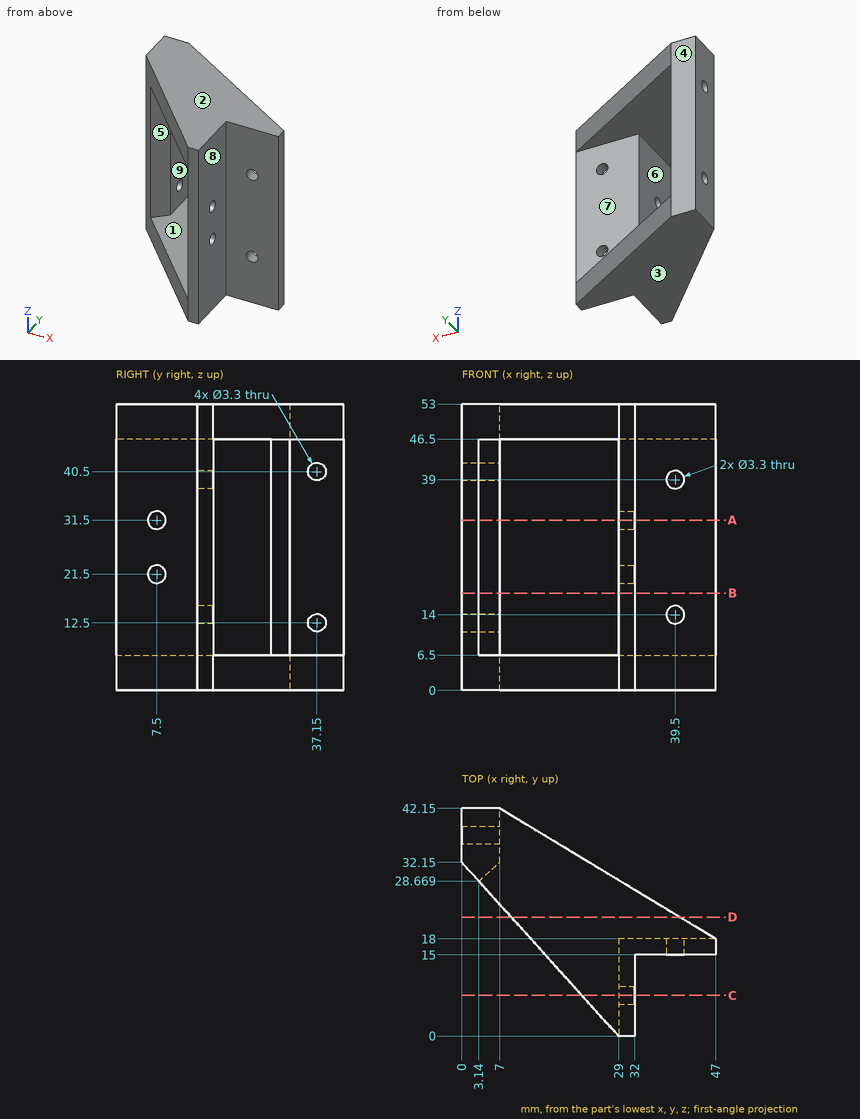
Study the drawing (mm; zero at the part's minimum x, y, z) and answer. A direction names the side the tool comes from. Give positions to 0.01 mm unless a question says otherwise; leave off trailing zeros. Loops run counter-clockwise (first coordinate to the right, second up) from the corner with the lowest first, then second, coordinate; pieces in that order, holes last. Notation, with made-up numbers: (83, 67) - (93, 67) arc R16 ccw to (93, 90) - close; hole circle Ø7 at (12, -40). An arc over 180 degrees is marked (long way). One line per question, with ' | ' between items.
(1) A tool of negligible diameter and unlimited length cuts with its end or side. For the marked faces 5, 6, 7, 8 and 9, from which of +Z, -Z, +X, -X, +Y, -Y can it reach the whole face along a straight path? Write none if from no direction.
Recorded:
face 5: +X, -Y | face 6: -X, +Y, -Y | face 7: +X, -X, +Y | face 8: +Z, -Z, +X, -Y | face 9: +X, +Y, -Y
(2) Each of these flat-tipped pins is pushed along its axis until it touches: pin 1 Ø2 at (y, z) = (37.15, 12.5) entering from -X; pin 2 Ø14.5 at (y, z) = (7, 24) entering from -X; pin 3 Ø20 at (x, z) = (42, 30.5) entering from +Y; pin 4 Ø5.5 at (x, z) = (39.5, 39) entering from -Y. Where does it stop, or does it pass through?
Recorded:
pin 1: passes through | pin 2: stops at x = 29 | pin 3: stops at y = 18 | pin 4: stops at y = 15
(3) The part is cut by section B-B (z = 18). Write down the section's boundary in (x, y).
Recorded:
outline: (0, 32.15) - (3.14, 28.67) - (7, 32.15) - (7, 42.15) - (0, 42.15) - close; (29, 0) - (32, 0) - (32, 15) - (47, 15) - (47, 18) - (29, 18) - close
(4) Straight lines are drawn through the part: probe 1 along Z at (x, y) = (25, 15); probe 2 along Z at (x, y) = (39.5, 15.6); probe 3 along Z at (x, y) = (29.75, 7.5). For each, find the intervals that lie inside material, in ascending order.
Recorded:
probe 1: z = 0 to 6.5, 46.5 to 53 | probe 2: z = 0 to 12.35, 15.65 to 37.35, 40.65 to 53 | probe 3: z = 0 to 19.85, 23.15 to 29.85, 33.15 to 53
(5) The mould has two halves that part along Z. Classify the marked faces 1, 2, 3 and 4: +Z half, -Z half, draft (parallel to the pull), parting line (faces both ways), or undercut.
Recorded:
face 1: undercut | face 2: +Z half | face 3: -Z half | face 4: draft
(6) The part is cut by section C-C (y = 7.5). Count the separate pieces of the cut face and the enclosed holes in it, then the cut area to 3 significant figures.
Recorded:
separate pieces: 3 | enclosed holes: 0 | area: 227 mm²
(7) The part is cut by section A-A (z = 31.5). Write down the section's boundary in (x, y).
Recorded:
outline: (0, 32.15) - (3.14, 28.67) - (7, 32.15) - (7, 42.15) - (0, 42.15) - close; (29, 0) - (32, 0) - (32, 5.85) - (29, 5.85) - close; (29, 9.15) - (32, 9.15) - (32, 15) - (47, 15) - (47, 18) - (29, 18) - close
(8) The part is cut by section D-D (y = 22). Write down the section's boundary in (x, z) (1 decimal), then the cut area to 3 significant figures.
Recorded:
outline: (9.2, 0) - (40.4, 0) - (40.4, 6.5) - (9.2, 6.5) - close; (9.2, 46.5) - (40.4, 46.5) - (40.4, 53) - (9.2, 53) - close | area: 406 mm²
